Input: dimensioned drawing with shaded views. Units: mm. Origin: part minimum x, y, z. A direction names the side the tool comes from. Give positions to 0.01 mm unless a question says otherwise; leave off trailing zeros. Write each loop counter-clockwise with the first axis right and the second up, starting at its lowest first coordinate (ties: lowest second). Pieces come first, ordered by that corner, then holes.
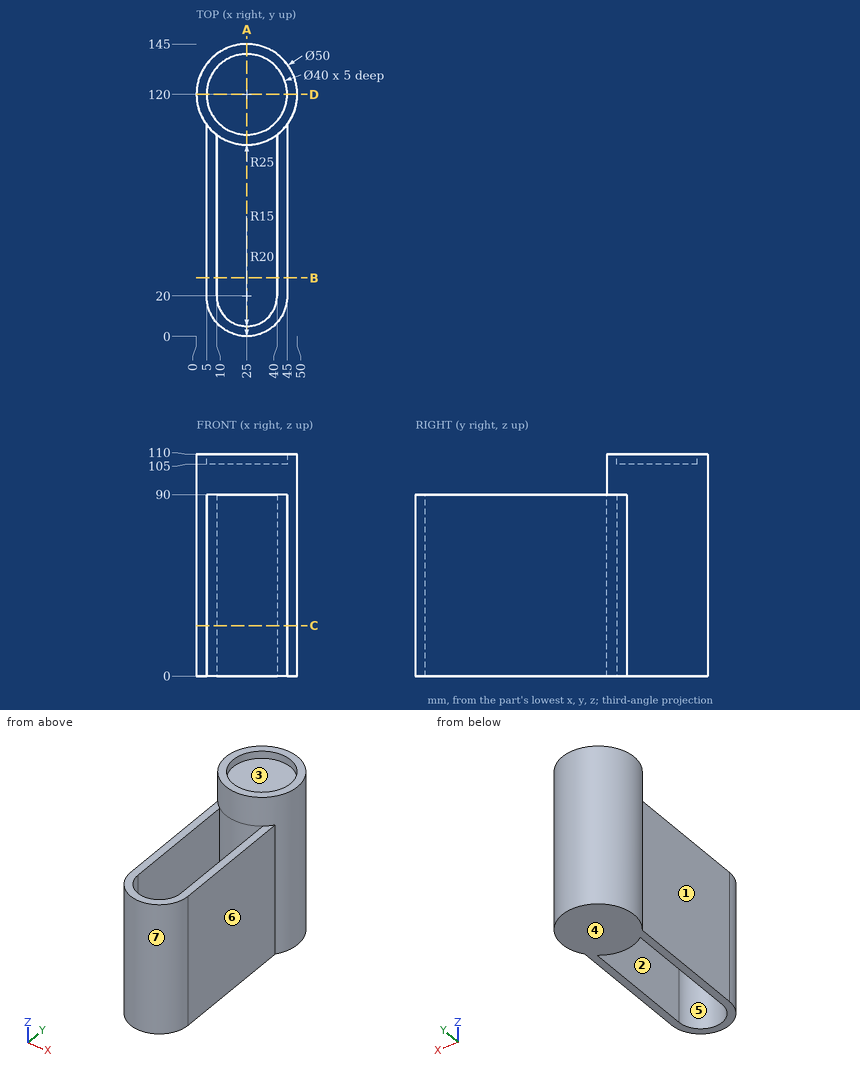
Item 1: Section C-C (z = 25). Return loops of the section in (x, y), and give its area (3 significant figures).
Item 2: Section A-A (x = 25). Return loops of the section in (y, z), and give its area (3 significant figures).
Item 3: Section B-B (y = 29). Return loops of the section in (x, z), and give its area (3 significant figures).
Item 4: Ray query, line 1 (X direction, y = 23.5, z = 26); line 2 (Y direction, x = 25, z = 107.35); line 3 (X direction, y = 10, z = 13). Return the intervals inside material, ascending.
Item 5: Set-up query: the marked faces 1, 2, 3 and 4. Return all of +Z, -Z, +X, -X, +Y, -Y with unobstructed straight access to the full face (end or side cutting, diameter ignored); none if empty.
Item 6: Mould query, pull axis Y, two halves, no side actions, for the marked faces 5, 6 and 7. Classes: +Y half, -Y half, draft (parallel to the pull), parting line (faces both ways), or undercut.
Item 7: Section D-D (y = 120). Return loops of the section in (x, z), and give its area (3 significant figures).
Item 8: Pin query (flat end, axial travel): pin 1 (8 mm diameter, centred on x = 9, z = 33.5, fed in from -Y); pin 2 (4 mm diameter, centred on x = 42, z = 51.5, fed in from -Y); pin 3 (2 mm diameter, centred on y = 126.5, z = 62.5, fed in from -X). Return the tip coordinate at first contact, or that it passes through.
Solved:
1. outline: (5, 20) arc R20 ccw to (45, 20) - (45, 105) arc R25 ccw (long way) to (5, 105) - close; hole (10, 20) arc R15 ccw to (40, 20) - (40, 100) arc R25 cw to (10, 100) - close
1. area: 3,060 mm2
2. outline: (0, 0) - (5, 0) - (5, 90) - (0, 90) - close; (95, 0) - (145, 0) - (145, 110) - (140, 110) - (140, 105) - (100, 105) - (100, 110) - (95, 110) - close
2. area: 5,750 mm2
3. outline: (5, 0) - (10, 0) - (10, 90) - (5, 90) - close; (40, 0) - (45, 0) - (45, 90) - (40, 90) - close
3. area: 900 mm2
4. line 1: x = 5 to 10, 40 to 45
4. line 2: y = 95 to 100, 140 to 145
4. line 3: x = 7.68 to 13.82, 36.18 to 42.32
5. face 1: +Z, -Z, -X, -Y
5. face 2: +Z, -Z
5. face 3: +Z
5. face 4: -Z, +X, -X, +Y, -Y
6. face 5: undercut
6. face 6: draft
6. face 7: -Y half
7. outline: (0, 0) - (50, 0) - (50, 110) - (45, 110) - (45, 105) - (5, 105) - (5, 110) - (0, 110) - close
7. area: 5,300 mm2
8. pin 1: stops at y = 4
8. pin 2: stops at y = 6.77
8. pin 3: stops at x = 0.61
